The model under review builds one solid part; all positions refer to its coordinate system, in mm. A direction names the side the tool comes from. Coordinates: 2 decimals unless noted, no trailing zeros. Order: outer loops, then holes, each group sorted by start corner. A loop starts at its lowest first (then second) coordinate and runs counter-clockwise, first axis right, second up. Notation, with made-up numbers: M 61,31.5 L 88,31.5 A25 ccw 88,58.5 Z; hole C -7,37.25 d3. An arc over 180 degrees is marked long. One line per item, written item: value.
```python
from build123d import *

# Parameters (mm, degrees)
BASE_FLANGE1_DEPTH    = 38.1
TAB1_DEPTH            = 3.175
EDGE_FLANGE1_DEPTH    = 50.8
FILLET2_R             = 1.5875
M6X1_0_TAPPED_HOLE1_D = 5
EDGE_FLANGE2_DEPTH    = 46.0375
FILLET1_R             = 3.175


# Sheet-metal steps are written as plain solids
with BuildPart() as part:
    # Sketch1 → Base-Flange1 (new, symmetric)
    with BuildSketch(Plane.XY):
        with BuildLine():
            Line((0, 19.05), (0, 4.7625))
            ThreePointArc((0, 4.7625), (1.394903955, 1.394903955), (4.7625, 0))
            Line((4.7625, 0), (50.8, 0))
            Line((50.8, 0), (50.8, 3.175))
            Line((50.8, 3.175), (4.7625, 3.175))
            ThreePointArc((4.7625, 3.175), (3.639967985, 3.639967985), (3.175, 4.7625))
            Line((3.175, 4.7625), (3.175, 19.05))
            Line((3.175, 19.05), (0, 19.05))
        make_face()
    extrude(amount=BASE_FLANGE1_DEPTH, both=True)

    # Sketch2 → Tab1 (add)
    with BuildSketch(Plane.XZ):
        Polygon((50.8, 38.1), (4.7625, 38.1), (4.7625, 41.275), (0, 41.275), (0, 63.5), (50.8, 63.5), align=None)
    extrude(amount=-TAB1_DEPTH)

    # Edge-Flange1 section (across the edge) → Edge-Flange1 (add)
    with BuildSketch(Plane(origin=(0, 3.175, 63.925369343), x_dir=(0, 0.8660254037844416, -0.49999999999999495), z_dir=(1, 0, 0))):
        with BuildLine():
            Line((-3.175, 0.425369343), (-3.175, 24.549261314))
            Line((-3.175, 24.549261314), (0, 24.549261314))
            Line((0, 24.549261314), (0, 0.425369343))
            ThreePointArc((0, 0.425369343), (0.054092751, 0.014494109), (0.212684671, -0.368380657))
            Line((0.212684671, -0.368380657), (-2.536945986, -1.955880657))
            ThreePointArc((-2.536945986, -1.955880657), (-3.012721748, -0.807256359), (-3.175, 0.425369343))
        make_face()
    extrude(amount=EDGE_FLANGE1_DEPTH)

    # Fillet2
    fillet2_edges = [part.edges().sort_by_distance(p)[0] for p in [
        (4.7625, 1.5875, 41.275),
        (0, 1.5875, 41.275),
    ]]
    fillet(fillet2_edges, radius=FILLET2_R)

    # M6x1.0 Tapped Hole1 (through all)
    with Locations(Plane(origin=(3.175, 0, 0), x_dir=(0, 0, -1), z_dir=(1, 0, 0))):
        with Locations((-25.4, 12.7), (25.4, 12.7)):
            Hole(M6X1_0_TAPPED_HOLE1_D / 2)

    # Edge-Flange2 section (across the edge) → Edge-Flange2 (add)
    with BuildSketch(Plane(origin=(50.8, 3.175, -39.6875), x_dir=(0, 0, 1), z_dir=(-1, 0, 0))):
        with BuildLine():
            Line((-3.175, 1.5875), (-3.175, 73.025))
            Line((-3.175, 73.025), (0, 73.025))
            Line((0, 73.025), (0, 1.5875))
            ThreePointArc((0, 1.5875), (0.464967985, 0.464967985), (1.5875, 0))
            Line((1.5875, 0), (1.5875, -3.175))
            ThreePointArc((1.5875, -3.175), (-1.780096045, -1.780096045), (-3.175, 1.5875))
        make_face()
    extrude(amount=EDGE_FLANGE2_DEPTH)

    # Fillet1
    fillet1_edges = [part.edges().sort_by_distance(p)[0] for p in [
        (4.7625, 76.2, -41.275),
        (1.5875, 19.05, 38.1),
        (0, 14.074815329, 85.979403285),
        (50.8, 14.074815329, 85.979403285),
        (1.5875, 19.05, -38.1),
        (50.8, 76.2, -41.275),
    ]]
    fillet(fillet1_edges, radius=FILLET1_R)


solid = part.part
```
(1) Tool access review of faces 1 (the flat face through (2, 8, 38.1)), 2 (the flat face through (25.044, 9.503, 74.886)), 3 (the flat face through (2, 8, -38.1)): name each direction out of +Z, -Z, +X, -X, +Y, -Y from which nothing blocks a thin tool from reaching the whole face with its end or side.
Geometry results:
face 1: -X, +Y, -Y
face 2: +X, -X, +Y
face 3: -Z, -X, +Y, -Y
(2) Insertion check: pin 1 Ø2.5 at (y, z) = (21, -41.5) entering from -X; pin 2 Ø1.5 at (x, z) = (24.5, -25) entering from +Y (3 decimals); pin 3 Ø1.5 at (x, y) = (18, 55) entering from +Z; pin 4 Ø3 at (y, z) = (12.7, -25.4) entering from +X. Each pin has a flat end and moves straight along its axis. Give the tip position at first contact, or say it passes through.
Geometry results:
pin 1: stops at x = 4.76
pin 2: stops at y = 3.175
pin 3: stops at z = -39.69
pin 4: passes through
(3) For L1, parallel to Z at x = 2, y = 12; L2, parallel to Z at x = 14.5, y = 30; L3, parallel to X at y = 8, z = -6 (3 decimals), list the stretches that pass through material, from the lowest coordinate up.
Geometry results:
L1: z = -38.1 to -27.8, -23 to 23, 27.8 to 38.1, 79.21 to 85.56
L2: z = -42.86 to -39.69
L3: x = 0 to 3.175
(4) We need section B-B, the plane x = 25. State the section outline as (y, z) points (1 decimal), plus the area to 3 significant figures.
Geometry results:
outline: M 0,-38.1 A4.8 ccw 4.8,-42.9 L 76.2,-42.9 L 76.2,-39.7 L 4.8,-39.7 A1.6 cw 3.2,-38.1 L 3.2,63.5 A1.6 cw 3.4,64.3 L 15.4,85.2 L 12.7,86.8 L 0.6,65.9 A4.8 ccw 0,63.5 Z
area: 647 mm2
(5) Mouldability with a two-part tool opening along Y and no side actions: class faces 4 (the flat face through (28, 76.2, -41)), 5 (the cylindrical face through (1.57, 14.81, -24.06)), 6 (the flat face through (50.8, 2, -7)) as +Y half, -Y half, draft (parallel to the pull), parting line (faces both ways), or undercut.
Geometry results:
face 4: +Y half
face 5: undercut
face 6: draft
(6) We need section D-D, the plane y = 63. State the section outline as (x, z) points.
Geometry results:
outline: M 4.76,-42.86 L 50.8,-42.86 L 50.8,-39.69 L 4.76,-39.69 Z
